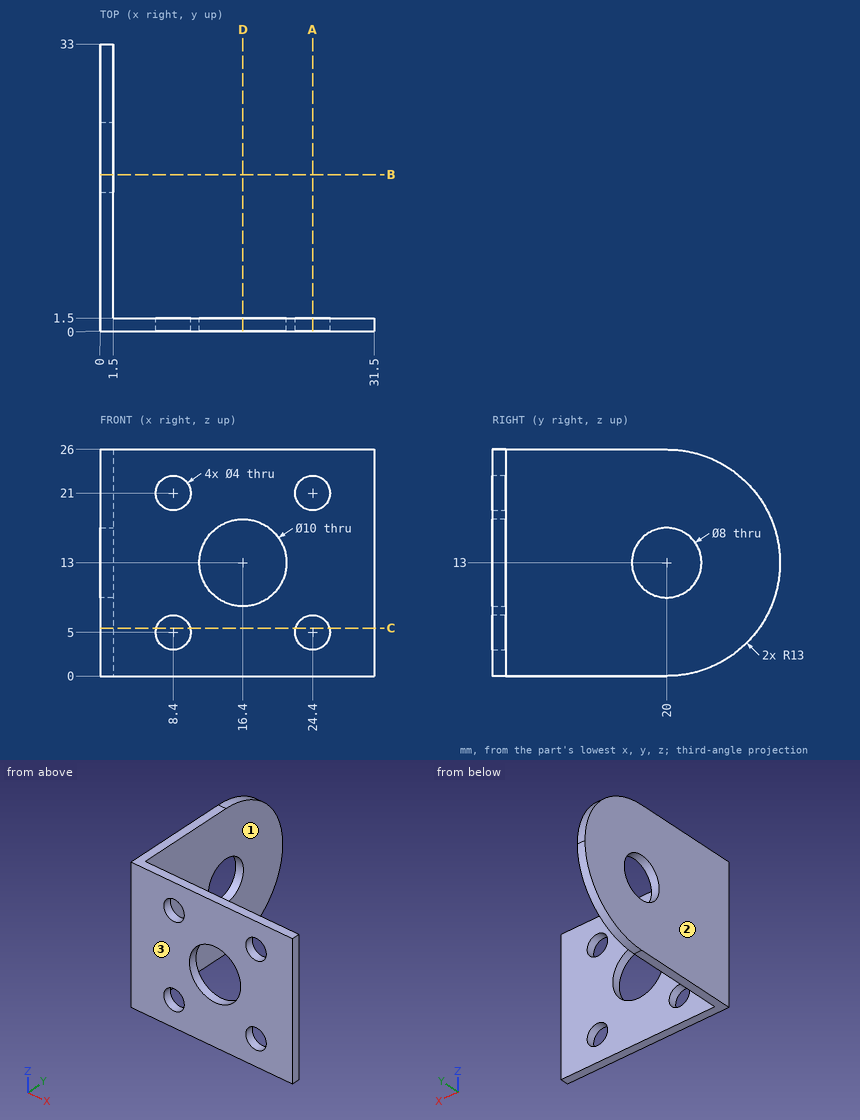
Design review of the part shown in the three views and the two pictorial views. Dimensions are in mm from the part's minimum x, y and z. Round coordinates to 2 decimals unless told otherwise and drop trailing zeros. Loops run counter-clockwise (first coordinate to the right, second up) from the corner with the lowest first, then second, coordinate; pieces in that order, holes last. Notation, with made-up numbers: (-13, 27) - (13, 27) arc R8 cw to (13, 35) - close; hole circle Ø6 at (38.25, 14.25). An arc over 180 degrees is marked (long way). One line per item, written item: value. Start each with the question number.
Item 1: Take a section at C-C (z = 5.5). Give the boundary of the cut face in (x, y).
Item 2: Clearance check with flat-ended pins moving along their axes: pin 1 Ø3.5 at (x, z) = (8.4, 5) entering from -Y; pin 2 Ø1.5 at (y, z) = (3.5, 21.5) entering from +X; pin 3 Ø10 at (x, z) = (17.5, 13) entering from +Y. State where each tip first meets the part, or that it passes through.
Item 3: Take a section at D-D (x = 16.4). Give the boundary of the cut face in (y, z), plus the area to 3 significant figures.
Item 4: Take a section at B-B (y = 18). Give the boundary of the cut face in (x, z), plus the area to 3 significant figures.
Item 5: The part is to be moulded in two halves that separate along X. For the marked faces 1, 2 and 3, say which applies: +X half, -X half, draft (parallel to the pull), parting line (faces both ways), or undercut.
Item 6: Take a section at A-A (x = 24.4). Give the boundary of the cut face in (y, z).
Item 7: For L1, parallel to X at y = 0.7, z = 5; L2, parallel to X at y = 0.65, z = 13; L3, parallel to Z at x = 24, y = 1, list the stretches that pass through material, from the lowest coordinate up.
Answer below:
1. outline: (0, 0) - (6.46, 0) - (6.46, 1.5) - (1.5, 1.5) - (1.5, 30.62) - (0, 30.62) - close; (10.34, 0) - (22.46, 0) - (22.46, 1.5) - (10.34, 1.5) - close; (26.34, 0) - (31.5, 0) - (31.5, 1.5) - (26.34, 1.5) - close
2. pin 1: passes through
2. pin 2: stops at x = 1.5
2. pin 3: stops at y = 1.5
3. outline: (0, 0) - (1.5, 0) - (1.5, 8) - (0, 8) - close; (0, 18) - (1.5, 18) - (1.5, 26) - (0, 26) - close
3. area: 24.0 mm2
4. outline: (0, 0) - (1.5, 0) - (1.5, 9.54) - (0, 9.54) - close; (0, 16.46) - (1.5, 16.46) - (1.5, 26) - (0, 26) - close
4. area: 28.6 mm2
5. face 1: +X half
5. face 2: -X half
5. face 3: draft
6. outline: (0, 0) - (1.5, 0) - (1.5, 3) - (0, 3) - close; (0, 7) - (1.5, 7) - (1.5, 19) - (0, 19) - close; (0, 23) - (1.5, 23) - (1.5, 26) - (0, 26) - close
7. L1: x = 0 to 6.4, 10.4 to 22.4, 26.4 to 31.5
7. L2: x = 0 to 11.4, 21.4 to 31.5
7. L3: z = 0 to 3.04, 6.96 to 19.04, 22.96 to 26
